```python
from build123d import *

# Parameters (mm, degrees)
SKETCH_1_W          = 140
SKETCH_1_H          = 100
EXTRUDE_1_DEPTH     = 4
SKETCH_9_R          = 2.75
CUT_EXTRUDE_3_DEPTH = 8
CHAMFER_2_SIZE      = 2
SKETCH_11_W         = 40
SKETCH_11_H         = 50
CUT_EXTRUDE_5_DEPTH = 5
SKETCH_12_W         = 10
SKETCH_12_H         = 15
EXTRUDE_2_DEPTH     = 14
SKETCH_13_W         = 60
SKETCH_13_H         = 15
EXTRUDE_3_DEPTH     = 14
SKETCH_14_W         = 28
SKETCH_14_H         = 70
EXTRUDE_4_DEPTH     = 20
SKETCH_15_W         = 28
SKETCH_15_H         = 70
EXTRUDE_5_DEPTH     = 20
SKETCH_16_R         = 6.75
CUT_EXTRUDE_6_DEPTH = 20
EXTRUDE_6_DEPTH     = 10
SKETCH_18_R         = 2.75
CUT_EXTRUDE_7_DEPTH = 96.268042911
SKETCH_19_R         = 2.75
CUT_EXTRUDE_8_DEPTH = 100
CHAMFER_3_SIZE      = 0.5
EXTRUDE_7_DEPTH     = 20
EXTRUDE_8_DEPTH     = 20
EXTRUDE_9_DEPTH     = 60
EXTRUDE_10_DEPTH    = 30
CHAMFER_4_SIZE      = 0.5
CHAMFER_5_SIZE      = 2
CHAMFER_6_SIZE      = 2
CHAMFER_7_SIZE      = 1
CUT_EXTRUDE_9_DEPTH = 100.564049794
CHAMFER_8_SIZE      = 4


with BuildPart() as part:
    # 草图1 → 凸台-拉伸1 (new body)
    with BuildSketch(Plane(origin=(0, 0, 0), x_dir=(0, 0, -1), z_dir=(1, 0, 0))):
        with Locations((0, -10)):
            Rectangle(SKETCH_1_W, SKETCH_1_H)
    extrude(amount=EXTRUDE_1_DEPTH)

    # 草图9 → 切除-拉伸3 (cut)
    with BuildSketch(Plane(origin=(4, 0, 0), x_dir=(0, 0, -1), z_dir=(1, 0, 0))):
        with Locations((-60, 20)):
            Circle(SKETCH_9_R)
        with Locations((60, 20)):
            Circle(SKETCH_9_R)
        with Locations((-45, -40)):
            Circle(SKETCH_9_R)
        with Locations((45, -40)):
            Circle(SKETCH_9_R)
    extrude(amount=-CUT_EXTRUDE_3_DEPTH, mode=Mode.SUBTRACT)

    # 倒角2
    chamfer_2_edges = [part.edges().sort_by_distance(p)[0] for p in [
        (2, 40, 70),
        (2, 40, -70),
        (2, -60, -70),
        (2, -60, 70),
    ]]
    chamfer(chamfer_2_edges, length=CHAMFER_2_SIZE)

    # 草图11 → 切除-拉伸5 (cut)
    with BuildSketch(Plane(origin=(4, 0, 0), x_dir=(0, 0, -1), z_dir=(1, 0, 0))):
        with Locations((0, 15)):
            Rectangle(SKETCH_11_W, SKETCH_11_H)
    extrude(amount=-CUT_EXTRUDE_5_DEPTH, mode=Mode.SUBTRACT)

    # 草图12 → 凸台-拉伸2 (add)
    with BuildSketch(Plane(origin=(4, 0, 0), x_dir=(0, 0, -1), z_dir=(1, 0, 0))):
        with Locations((-25, 32.5)):
            Rectangle(SKETCH_12_W, SKETCH_12_H)
        with Locations((25, 32.5)):
            Rectangle(SKETCH_12_W, SKETCH_12_H)
    extrude(amount=EXTRUDE_2_DEPTH)

    # 草图13 → 凸台-拉伸3 (add)
    with BuildSketch(Plane(origin=(18, 0, 0), x_dir=(0, 0, -1), z_dir=(1, 0, 0))):
        with Locations((0, 32.5)):
            Rectangle(SKETCH_13_W, SKETCH_13_H)
    extrude(amount=EXTRUDE_3_DEPTH)

    # 草图14 → 凸台-拉伸4 (add)
    with BuildSketch(Plane.XY.offset(30)):
        with Locations((18, 5)):
            Rectangle(SKETCH_14_W, SKETCH_14_H)
    extrude(amount=EXTRUDE_4_DEPTH)

    # 草图15 → 凸台-拉伸5 (add)
    with BuildSketch(Plane(origin=(0, 0, -30), x_dir=(-1, 0, 0), z_dir=(0, 0, -1))):
        with Locations((-18, 5)):
            Rectangle(SKETCH_15_W, SKETCH_15_H)
    extrude(amount=EXTRUDE_5_DEPTH)

    # 草图16 → 切除-拉伸6 (cut)
    with BuildSketch(Plane(origin=(0, 40, 0), x_dir=(1, 0, 0), z_dir=(0, 1, 0))):
        with Locations((18, 0)):
            Circle(SKETCH_16_R)
    extrude(amount=-CUT_EXTRUDE_6_DEPTH, mode=Mode.SUBTRACT)

    # 草图17 → 凸台-拉伸6 (add)
    with BuildSketch(Plane(origin=(32, 0, 0), x_dir=(0, 0, -1), z_dir=(1, 0, 0))):
        Polygon((50, 40), (-50, 40), (-50, -30), (-30, -30), (-30, 25), (30, 25), (30, -30), (50, -30), align=None)
    extrude(amount=EXTRUDE_6_DEPTH)

    # 草图18 → 切除-拉伸7 (cut, through all)
    with BuildSketch(Plane.ZY.offset(-18)):
        with Locations((14, 32.5)):
            Circle(SKETCH_18_R)
        with Locations((-14, 32.5)):
            Circle(SKETCH_18_R)
    extrude(amount=-CUT_EXTRUDE_7_DEPTH, mode=Mode.SUBTRACT)

    # 草图19 → 切除-拉伸8 (cut)
    with BuildSketch(Plane(origin=(42, 0, 0), x_dir=(0, 0, -1), z_dir=(1, 0, 0))):
        with Locations((0, 32.5)):
            Circle(SKETCH_19_R)
    extrude(amount=-CUT_EXTRUDE_8_DEPTH, mode=Mode.SUBTRACT)

    # 倒角3
    chamfer_3_edges = [part.edges().sort_by_distance(p)[0] for p in [
        (4, 20, 62.75),
        (4, -40, -42.25),
        (4, -40, 47.75),
        (4, 20, -57.25),
    ]]
    chamfer(chamfer_3_edges, length=CHAMFER_3_SIZE)

    # 草图20 → 凸台-拉伸7 (add)
    with BuildSketch(Plane.XY.offset(50)):
        Polygon((42, 25), (4, -30), (32, 25), align=None)
    extrude(amount=-EXTRUDE_7_DEPTH)

    # 草图21 → 凸台-拉伸8 (add)
    with BuildSketch(Plane(origin=(0, 0, -50), x_dir=(-1, 0, 0), z_dir=(0, 0, -1))):
        Polygon((-42, 25), (-4, -30), (-32, 25), align=None)
    extrude(amount=-EXTRUDE_8_DEPTH)

    # 草图22 → 凸台-拉伸9 (add)
    with BuildSketch(Plane.XY.offset(-30)):
        Polygon((42, -17), (4, -17), (4, -60), (42, -30), align=None)
    extrude(amount=EXTRUDE_9_DEPTH)

    # 草图23 → 凸台-拉伸10 (add)
    with BuildSketch(Plane.XZ.offset(30)):
        Polygon((42, 50), (4, 70), (4, 50), align=None)
    extrude_10 = extrude(amount=-EXTRUDE_10_DEPTH)

    # 镜向1: 凸台-拉伸10 across plane
    add(extrude_10.mirror(Plane.XY))

    # 倒角4
    chamfer_4_edges = [part.edges().sort_by_distance(p)[0] for p in [
        (42, 32.5, 11.25),
        (42, 32.5, -16.75),
        (42, 32.5, 2.75),
    ]]
    chamfer(chamfer_4_edges, length=CHAMFER_4_SIZE)

    # 倒角5
    chamfer_5_edges = [part.edges().sort_by_distance(p)[0] for p in [
        (42, 25, 0),
        (42, 4, -30),
        (42, 4, 30),
        (42, -17, 0),
    ]]
    chamfer(chamfer_5_edges, length=CHAMFER_5_SIZE)

    # 倒角6
    chamfer_6_edges = [part.edges().sort_by_distance(p)[0] for p in [
        (42, -30, 40),
        (42, -30, -40),
        (42, 20, 50),
        (42, 20, -50),
        (23, 40, -50),
        (42, 40, 0),
        (23, 40, 50),
    ]]
    chamfer(chamfer_6_edges, length=CHAMFER_6_SIZE)

    # 倒角7
    chamfer_7_edges = [part.edges().sort_by_distance(p)[0] for p in [
        (0, -10, 0),
        (0, 15, -20),
        (0, 15, 20),
    ]]
    chamfer(chamfer_7_edges, length=CHAMFER_7_SIZE)

    # 草图24 → 切除-拉伸9 (cut, through all)
    with BuildSketch(Plane(origin=(0, -17, 0), x_dir=(1, 0, 0), z_dir=(0, 1, 0))):
        with BuildLine():
            Line((28, 6.75), (43.669106449, 6.75))
            Line((43.669106449, 6.75), (43.669106449, -6.75))
            Line((43.669106449, -6.75), (28, -6.75))
            ThreePointArc((28, -6.75), (21.25, 0), (28, 6.75))
        make_face()
    extrude(amount=-CUT_EXTRUDE_9_DEPTH, mode=Mode.SUBTRACT)

    # 倒角8
    chamfer_8_edges = [part.edges().sort_by_distance(p)[0] for p in [
        (34, -17, -6.75),
        (34, -17, 6.75),
        (21.25, -17, 0),
    ]]
    chamfer(chamfer_8_edges, length=CHAMFER_8_SIZE)


solid = part.part
```
Input: part model. Units: mm. Frame: model coordinates. A direction names the side the tool comes from. Coordinates: 2 decimals unless noted, no trailing zeros. Write each loop counter-clockwise with the first axis right and the second up, starting at its lowest first coordinate (ties: lowest second). Pieces come first, ordered by that corner, then holes. Notation, with made-up numbers: (-21.75, 68.25) -> (12.25, 68.25) arc R25 ccw to (12.25, 98.25) -> close; hole circle Ø7 at (29, 87.25). An arc over 180 degrees is marked (long way). Write each question's results on one line, items separated by ' | '.
Item 1: Section query A-A on y = 20. Count the separate pieces of the cut face and the enclosed holes in it, plus the area to 3 significant figures.
Conclusion:
separate pieces: 4 | enclosed holes: 0 | area: 1,870 mm^2
Item 2: Pin query (flat end, axial travel): pin 1 Ø6.5 at (y, z) = (33.5, -11) entering from -X; pin 2 Ø0.9 at (x, z) = (2.5, 2.5) entering from +Y; pin 3 Ø9.5 at (x, y) = (28, -39.5) entering from +Z. Return the tip coordinate at first contact, or that it passes through.
Conclusion:
pin 1: stops at x = 18 | pin 2: stops at y = -10 | pin 3: stops at z = 30
Item 3: Section query B-B on z = 0. Return loops of the section in (x, y).
Conclusion:
outline: (0, -60) -> (4, -60) -> (21.25, -46.38) -> (21.25, -21) -> (17.25, -17) -> (4, -17) -> (4, -10) -> (1, -10) -> (0, -11) -> close; (24.75, 25) -> (40, 25) -> (42, 27) -> (42, 29.25) -> (41.5, 29.75) -> (24.75, 29.75) -> close; (24.75, 35.25) -> (41.5, 35.25) -> (42, 35.75) -> (42, 38) -> (40, 40) -> (24.75, 40) -> close
Item 4: Section query D-D on x = 31. Return loops of the section in (y, z), plus the area to 3 significant figures.
Conclusion:
outline: (-38.68, -30) -> (-30, -30) -> (-30, -55.79) -> (0, -55.79) -> (0, -50) -> (38, -50) -> (40, -48) -> (40, 48) -> (38, 50) -> (0, 50) -> (0, 55.79) -> (-30, 55.79) -> (-30, 30) -> (-38.68, 30) -> (-38.68, 6.75) -> (-21, 6.75) -> (-17, 10.75) -> (-17, 30) -> (25, 30) -> (25, -30) -> (-17, -30) -> (-17, -10.75) -> (-21, -6.75) -> (-38.68, -6.75) -> close; hole circle Ø5.5 at (32.5, -14); hole circle Ø5.5 at (32.5, 0); hole circle Ø5.5 at (32.5, 14) | area: 4,960 mm^2
Item 5: Material intervals for probe 1 along Y at (x, z) = (1.8, -60); probe 2 along Z at (x, y) = (32.5, 0.5); probe 3 along Y at (x, z) = (29, 0), sorted ascending.
Conclusion:
probe 1: y = -60 to 17.25, 22.75 to 40 | probe 2: z = -50 to -30, 30 to 50 | probe 3: y = 25 to 29.75, 35.25 to 40
Item 6: Section query C-C on z = 60. Return loops of the section in (x, y).
Conclusion:
outline: (0, -60) -> (4, -60) -> (4, -30) -> (23, -30) -> (23, 0) -> (4, 0) -> (4, 16.75) -> (3.5, 17.25) -> (0, 17.25) -> close; (0, 22.75) -> (3.5, 22.75) -> (4, 23.25) -> (4, 40) -> (0, 40) -> close
Item 7: Mould query, pull axis Z, two halves, no side actions, for faces 4 (the flat face through (4, 20, -64)), 5 (the flat face through (23, -15, 60)), 6 (the flat face through (8, 26, -20)). Classes: +Z half, -Z half, draft (parallel to the pull), parting line (faces both ways), or undercut.
Conclusion:
face 4: draft | face 5: +Z half | face 6: undercut
Item 8: Set-up query: faces 1 (the flat face through (18, 33, 11)), 2 (the flat face through (22, 19, 50)), 3 (the flat face through (34.9, -19.03, -8.72)). Return all of +Z, -Z, +X, -X, +Y, -Y with unobstructed straight access to the full face (end or side cutting, diameter ignored); none if empty.
Conclusion:
face 1: -X, +Y | face 2: +Z, +X, +Y | face 3: +X
